```python
from build123d import *

# Parameters (mm, degrees)
SKETCH1_W                = 20
SKETCH1_H                = 10
BOSS_EXTRUDE1_DEPTH      = 3
SKETCH2_W                = 8
SKETCH2_H                = 9.5
BOSS_EXTRUDE2_DEPTH      = 6
BOSS_EXTRUDE3_DEPTH      = 6
BOSS_EXTRUDE3_DEPTH_BACK = 1.5
SKETCH3_R                = 6
CHAMFER1_SIZE            = 1
CHAMFER2_SIZE            = 1
CHAMFER3_SIZE            = 1
CHAMFER4_SIZE            = 2
CHAMFER5_SIZE            = 2
M2_CLEARANCE_HOLE1_D     = 2.4
SKETCH21_R               = 4.075
CUT_EXTRUDE10_DEPTH      = 6.5
SKETCH25_W               = 12
SKETCH25_H               = 4.5
BOSS_EXTRUDE6_DEPTH      = 3
M1_6_TAPPED_HOLE2_D      = 1.25
CUT_EXTRUDE15_START      = -3
SKETCH40_R               = 6
CUT_EXTRUDE15_DEPTH      = 3
BOSS_EXTRUDE8_START      = 1.7
SKETCH41_R               = 5
SKETCH41_R_2             = 4.075
BOSS_EXTRUDE8_DEPTH      = 1.7
CUT_EXTRUDE16_DEPTH      = 1


with BuildPart() as part:
    # Sketch1 → Boss-Extrude1 (new body)
    with BuildSketch(Plane.XY):
        Rectangle(SKETCH1_W, SKETCH1_H)
    extrude(amount=BOSS_EXTRUDE1_DEPTH)

    # Sketch2 → Boss-Extrude2 (add)
    with BuildSketch(Plane(origin=(0, 0, 0), x_dir=(-1, 0, 0), z_dir=(0, 0, -1))):
        with Locations((0, 4.75)):
            Rectangle(SKETCH2_W, SKETCH2_H)
    extrude(amount=BOSS_EXTRUDE2_DEPTH)

    # Sketch3 → Boss-Extrude3 (add, two sides: drawn at the far end of the back side and taken through both)
    with BuildSketch(Plane(origin=(0, 0, -6), x_dir=(-1, 0, 0), z_dir=(0, 0, -1)).offset(-BOSS_EXTRUDE3_DEPTH_BACK)):
        with Locations((0, 8.25)):
            Circle(SKETCH3_R)
    extrude(amount=BOSS_EXTRUDE3_DEPTH + BOSS_EXTRUDE3_DEPTH_BACK)

    # Chamfer1
    chamfer1_edges = [part.edges().sort_by_distance(p)[0] for p in [
        (-10, 5, 1.5),
        (10, 5, 1.5),
        (10, -5, 1.5),
        (-10, -5, 1.5),
    ]]
    chamfer(chamfer1_edges, length=CHAMFER1_SIZE)

    # Chamfer2
    chamfer2_edges = [part.edges().sort_by_distance(p)[0] for p in [
        (4, 2.5, 0),
        (-4, 2.5, 0),
        (0, 0, 0),
        (0, 0, -6),
    ]]
    chamfer(chamfer2_edges, length=CHAMFER2_SIZE)

    # Chamfer3
    # the kernel refuses this chamfer: 1 mm, written as the material it adds along each edge
    with BuildSketch(Plane(origin=(0, 8.25, -6), x_dir=(0.9161991076005935, -0.4007233400138756, 0), z_dir=(0.4007233400138756, 0.9161991076005935, 0))) as chamfer3_piece_1_section:
        Polygon((6 + CHAMFER3_SIZE, 0), (6, CHAMFER3_SIZE), (6, 0), align=None)
    chamfer3_piece_1 = revolve(axis=Axis((0, 8.25, -6), (0, 0, -1)), revolution_arc=132.753188511, mode=Mode.PRIVATE)
    chamfer3_piece_1 = split(chamfer3_piece_1, bisect_by=Plane(origin=(-4, 1.761901104, -6.488098896), z_dir=(1, 0, 0)), keep=Keep.TOP, mode=Mode.PRIVATE)
    chamfer3_piece_1 = split(chamfer3_piece_1, bisect_by=Plane(origin=(4, 1.761901104, -6.488098896), z_dir=(-1, 0, 0)), keep=Keep.TOP, mode=Mode.PRIVATE)
    add(chamfer3_piece_1)

    # Chamfer4
    chamfer4_edges = [part.edges().sort_by_distance(p)[0] for p in [
        (0, 5, 0),
    ]]
    chamfer(chamfer4_edges, length=CHAMFER4_SIZE)

    # Chamfer5
    # the kernel refuses this chamfer: 2 mm, written as the material it adds along each edge
    with BuildSketch(Plane(origin=(4, 5, -6.143365976), x_dir=(0.9996219169112968, -0.02749587661058651, 0), z_dir=(0, 0, 1))) as chamfer5_piece_1_section:
        Polygon((CHAMFER5_SIZE * 0.999621916911, CHAMFER5_SIZE * 0.0274958766106), (-CHAMFER5_SIZE * 0.0274958766106, CHAMFER5_SIZE * 0.999621916911), (0, 0), align=None)
    chamfer5_piece_1 = extrude(amount=13.286731952, mode=Mode.PRIVATE)
    chamfer5_piece_1 = split(chamfer5_piece_1, bisect_by=Plane(origin=(4.448565439, 5.872663391, -0.551434561), z_dir=(-0.7071067811865476, 0, 0.7071067811865476)), keep=Keep.TOP, mode=Mode.PRIVATE)
    chamfer5_piece_1 = split(chamfer5_piece_1, bisect_by=Plane(origin=(4.264786899, 6.620159706, 0.379840294), z_dir=(0, -0.7071067811865476, -0.7071067811865476)), keep=Keep.TOP, mode=Mode.PRIVATE)
    chamfer5_piece_1 = split(chamfer5_piece_1, bisect_by=Plane(origin=(4.264786899, 5.872663391, 0), z_dir=(0, 0, -1)), keep=Keep.TOP, mode=Mode.PRIVATE)
    add(chamfer5_piece_1)
    with BuildSketch(Plane(origin=(4, 5, -6.143365976), x_dir=(0.9996219169112968, -0.02749587661058651, 0), z_dir=(0, 0, 1))) as chamfer5_piece_2_section:
        Polygon((CHAMFER5_SIZE * 0.999621916911, CHAMFER5_SIZE * 0.0274958766106), (-CHAMFER5_SIZE * 0.0274958766106, CHAMFER5_SIZE * 0.999621916911), (0, 0), align=None)
    chamfer5_piece_2 = extrude(amount=13.286731952, mode=Mode.PRIVATE)
    chamfer5_piece_2 = split(chamfer5_piece_2, bisect_by=Plane(origin=(5.409489173, 5.195513982, 0.409489173), z_dir=(0.7071067811865476, 0, -0.7071067811865476)), keep=Keep.TOP, mode=Mode.PRIVATE)
    chamfer5_piece_2 = split(chamfer5_piece_2, bisect_by=Plane(origin=(5.545985564, 5.195513982, 0), z_dir=(0, 0, 1)), keep=Keep.TOP, mode=Mode.PRIVATE)
    add(chamfer5_piece_2)
    with BuildSketch(Plane(origin=(4, 5, -6.143365976), x_dir=(0.9996219169112968, -0.02749587661058651, 0), z_dir=(0, 0, 1))) as chamfer5_piece_3_section:
        Polygon((CHAMFER5_SIZE * 0.999621916911, CHAMFER5_SIZE * 0.0274958766106), (-CHAMFER5_SIZE * 0.0274958766106, CHAMFER5_SIZE * 0.999621916911), (0, 0), align=None)
    chamfer5_piece_3 = extrude(amount=13.286731952, mode=Mode.PRIVATE)
    chamfer5_piece_3 = split(chamfer5_piece_3, bisect_by=Plane(origin=(5.251928591, 5.490690976, 0.251928591), z_dir=(-0.7071067811865476, 0, 0.7071067811865476)), keep=Keep.TOP, mode=Mode.PRIVATE)
    chamfer5_piece_3 = split(chamfer5_piece_3, bisect_by=Plane(origin=(4.702100532, 5.844467162, 1.155532838), z_dir=(0, -0.7071067811865476, -0.7071067811865476)), keep=Keep.TOP, mode=Mode.PRIVATE)
    chamfer5_piece_3 = split(chamfer5_piece_3, bisect_by=Plane(origin=(4.702100532, 5.490690976, 0), z_dir=(0, 0, 1)), keep=Keep.TOP, mode=Mode.PRIVATE)
    add(chamfer5_piece_3)
    with BuildSketch(Plane(origin=(-4, 5, 7.143365976), x_dir=(-0.9996219169112968, -0.027495876610586487, 0), z_dir=(0, 0, -1))) as chamfer5_piece_4_section:
        Polygon((CHAMFER5_SIZE * 0.999621916911, CHAMFER5_SIZE * 0.0274958766106), (-CHAMFER5_SIZE * 0.0274958766106, CHAMFER5_SIZE * 0.999621916911), (0, 0), align=None)
    chamfer5_piece_4 = extrude(amount=13.286731952, mode=Mode.PRIVATE)
    chamfer5_piece_4 = split(chamfer5_piece_4, bisect_by=Plane(origin=(-5.251928591, 5.490690976, 0.251928591), z_dir=(0.7071067811865476, 0, 0.7071067811865476)), keep=Keep.TOP, mode=Mode.PRIVATE)
    chamfer5_piece_4 = split(chamfer5_piece_4, bisect_by=Plane(origin=(-4.702100532, 5.844467162, 1.155532838), z_dir=(0, -0.7071067811865476, -0.7071067811865476)), keep=Keep.TOP, mode=Mode.PRIVATE)
    chamfer5_piece_4 = split(chamfer5_piece_4, bisect_by=Plane(origin=(-4.702100532, 5.490690976, 0), z_dir=(0, 0, 1)), keep=Keep.TOP, mode=Mode.PRIVATE)
    add(chamfer5_piece_4)
    with BuildSketch(Plane(origin=(-4, 5, 7.143365976), x_dir=(-0.9996219169112968, -0.027495876610586487, 0), z_dir=(0, 0, -1))) as chamfer5_piece_5_section:
        Polygon((CHAMFER5_SIZE * 0.999621916911, CHAMFER5_SIZE * 0.0274958766106), (-CHAMFER5_SIZE * 0.0274958766106, CHAMFER5_SIZE * 0.999621916911), (0, 0), align=None)
    chamfer5_piece_5 = extrude(amount=13.286731952, mode=Mode.PRIVATE)
    chamfer5_piece_5 = split(chamfer5_piece_5, bisect_by=Plane(origin=(-4.448565439, 5.872663391, -0.551434561), z_dir=(0.7071067811865476, 0, 0.7071067811865476)), keep=Keep.TOP, mode=Mode.PRIVATE)
    chamfer5_piece_5 = split(chamfer5_piece_5, bisect_by=Plane(origin=(-4.264786899, 6.620159706, 0.379840294), z_dir=(0, -0.7071067811865476, -0.7071067811865476)), keep=Keep.TOP, mode=Mode.PRIVATE)
    chamfer5_piece_5 = split(chamfer5_piece_5, bisect_by=Plane(origin=(-4.264786899, 5.872663391, 0), z_dir=(0, 0, -1)), keep=Keep.TOP, mode=Mode.PRIVATE)
    add(chamfer5_piece_5)
    with BuildSketch(Plane(origin=(-4, 5, 7.143365976), x_dir=(-0.9996219169112968, -0.027495876610586487, 0), z_dir=(0, 0, -1))) as chamfer5_piece_6_section:
        Polygon((CHAMFER5_SIZE * 0.999621916911, CHAMFER5_SIZE * 0.0274958766106), (-CHAMFER5_SIZE * 0.0274958766106, CHAMFER5_SIZE * 0.999621916911), (0, 0), align=None)
    chamfer5_piece_6 = extrude(amount=13.286731952, mode=Mode.PRIVATE)
    chamfer5_piece_6 = split(chamfer5_piece_6, bisect_by=Plane(origin=(-5.409489173, 5.195513982, 0.409489173), z_dir=(-0.7071067811865476, 0, -0.7071067811865476)), keep=Keep.TOP, mode=Mode.PRIVATE)
    chamfer5_piece_6 = split(chamfer5_piece_6, bisect_by=Plane(origin=(-5.545985564, 5.195513982, 0), z_dir=(0, 0, 1)), keep=Keep.TOP, mode=Mode.PRIVATE)
    add(chamfer5_piece_6)

    # M2 Clearance Hole1 (through all)
    with Locations(Plane(origin=(0, 0, 0), x_dir=(-1, 0, 0), z_dir=(0, 0, -1))):
        with Locations((8, -3), (-8, -3)):
            Hole(M2_CLEARANCE_HOLE1_D / 2)

    # Sketch21 → Cut-Extrude10 (cut)
    with BuildSketch(Plane(origin=(0, 0, -12), x_dir=(-1, 0, 0), z_dir=(0, 0, -1))):
        with Locations((0, 8.25)):
            Circle(SKETCH21_R)
    extrude(amount=-CUT_EXTRUDE10_DEPTH, mode=Mode.SUBTRACT)

    # Sketch25 → Boss-Extrude6 (add)
    with BuildSketch(Plane.XY):
        with Locations((0, 7.25)):
            Rectangle(SKETCH25_W, SKETCH25_H)
    extrude(amount=BOSS_EXTRUDE6_DEPTH)

    # Sketch24 → CSK SLOT for M1.6 Countersunk Flat Head (revolve, cut)
    with BuildSketch(Plane(origin=(0, 8.25, 3), x_dir=(0, -1, 0), z_dir=(1, 0, 0))):
        Polygon((0, 0), (0, 40.540774557), (0.9, 40), (0.9, 9.9), (1.8, 9), (1.8, 0), align=None)
    revolve(axis=Axis((0, 8.25, 9.35), (0, 0, -1)), mode=Mode.SUBTRACT)

    # M1.6 Tapped Hole2 (through all)
    with Locations(Plane.ZY.offset(6)):
        with Locations((-7, 8.25)):
            Hole(M1_6_TAPPED_HOLE2_D / 2)

    # Sketch40 → Cut-Extrude15 (cut)
    with BuildSketch(Plane(origin=(0, 0, -12), x_dir=(-1, 0, 0), z_dir=(0, 0, -1)).offset(CUT_EXTRUDE15_START)):
        with Locations((0, 8.25)):
            Circle(SKETCH40_R)
    extrude(amount=CUT_EXTRUDE15_DEPTH, mode=Mode.SUBTRACT)

    # Sketch41 → Boss-Extrude8 (add)
    with BuildSketch(Plane(origin=(0, 0, -9), x_dir=(-1, 0, 0), z_dir=(0, 0, -1)).offset(BOSS_EXTRUDE8_START)):
        with Locations((0, 8.25)):
            Circle(SKETCH41_R)
        with Locations((0, 8.25)):
            Circle(SKETCH41_R_2, mode=Mode.SUBTRACT)
    extrude(amount=-BOSS_EXTRUDE8_DEPTH)

    # Sketch43 → Cut-Extrude16 (cut)
    with BuildSketch(Plane.XY.offset(-4.5)):
        with BuildLine():
            Line((-4, 9.5), (-1.295183385, 9.5))
            ThreePointArc((-1.295183385, 9.5), (0, 10.05), (1.295183385, 9.5))
            Line((1.295183385, 9.5), (4, 9.5))
            Line((4, 9.5), (5.868347297, 9.5))
            ThreePointArc((5.868347297, 9.5), (0, 14.25), (-5.868347297, 9.5))
            Line((-5.868347297, 9.5), (-4, 9.5))
        make_face()
    extrude(amount=-CUT_EXTRUDE16_DEPTH, mode=Mode.SUBTRACT)


solid = part.part
```
Geometry check sheet. Reference: the model listing, model coordinates, mm. A direction names the side the tool comes from. Coordinates: 2 decimals unless noted, no trailing zeros. Loops run counter-clockwise (first coordinate to the right, second up) from the corner with the lowest first, then second, coordinate; pieces in that order, holes last.
Item 1: Thickness scan on line 1 (Z direction, x = -5.1, y = 8.25) (3 decimals); line 2 (Y direction, x = -8, z = 2.3); line 3 (X direction, y = 8.25, z = -8.4) (3 decimals). Record the ranges inside material, lowest first.
Item 2: Sectioned sample at A-A, the plane y = -3. Record the boundary of the cut face in (x, z).
Item 3: Release check for a two-part mould opening along Y. For faces 5 (the face through (6.8, -2.95, 1.52)), 6 (the face through (-8, 5, 1)), 7 (the face through (0.1, 0.5, -5.5)), 8 (the face through (5.027, 8.672, -6.539)) record: released by +Y, released by -Y, zero draft, split by the parting line, or undercut.
Item 4: Go/stop test with flat-tipped pins: pin 1 Ø3.5 at (y, z) = (6, -5) entering from +X; pin 2 Ø1.5 at (y, z) = (7.5, -5.5) entering from -X; pin 3 Ø4 at (x, z) = (-1.5, -7.5) entering from +Y; pin 4 Ø1.7 at (x, y) = (1.5, 2) entering from -Z. Record where each tip stops, or that it passes through.
Item 5: Sectioned sample at C-C, the plane z = -0.25. Record the boundary of the cut face in (x, y), then the cut area to 3 significant figures.
Item 6: Sectioned sample at D-D, the plane y = 6.75. Record the boundary of the cut face in (x, z), then the cut area to 3 significant figures.
Item 7: Sectioned sample at B-B, the plane x = 8. Record the boundary of the cut face in (y, z).
Item 8: Access from +Z, -Z, +X, -X, +Y, -Y to the whole of each face (thin tool, end or side, straight path). Record for faces 1 (the face through (-3.764, 6.689, -8.136)), 2 (the face through (0, 13, -5.5)), 3 (the face through (0, 0, -3)), 4 (the face through (7, 5, 1)).
Check result:
1. line 1: z = -9 to -7.625, -6.375 to -4.5, 0 to 3
1. line 2: y = -5 to -4.2, -1.8 to 5
1. line 3: x = -6 to -4.075, 4.075 to 6
2. outline: (-10, 0) - (-9.2, 0) - (-9.2, 3) - (-10, 3) - close; (-6.8, 0) - (6.8, 0) - (6.8, 3) - (-6.8, 3) - close; (9.2, 0) - (10, 0) - (10, 3) - (9.2, 3) - close
3. face 5: undercut
3. face 6: released by +Y
3. face 7: released by -Y
3. face 8: undercut
4. pin 1: stops at x = 5.98
4. pin 2: stops at x = -6
4. pin 3: stops at y = 14.25
4. pin 4: stops at z = -9
5. outline: (-4.75, -0.75) - (4.75, -0.75) - (4.75, 6.25) - (4, 7) - (4, 9.5) - (1.3, 9.5) arc R1.8 cw (long way) to (-1.3, 9.5) - (-4, 9.5) - (-4, 7) - (-4.75, 6.25) - close
5. area: 83.9 mm2
6. outline: (-6, 0) - (-4.25, 0) - (-4.25, -0.75) - (-4, -1) - (-4, -4.5) - (-5.81, -4.5) - (-5.81, -9) - (-4.77, -9) - (-4.77, -10.7) - (-3.79, -10.7) - (-3.79, -5.5) - (-0.99, -5.5) - (-0.99, 3) - (-6, 3) - close; (0.99, -5.5) - (3.79, -5.5) - (3.79, -10.7) - (4.77, -10.7) - (4.77, -9) - (5.81, -9) - (5.81, -4.5) - (4, -4.5) - (4, -1) - (4.25, -0.75) - (4.25, 0) - (6, 0) - (6, 3) - (0.99, 3) - close
6. area: 84.6 mm2
7. outline: (-5, 0) - (-4.2, 0) - (-4.2, 3) - (-5, 3) - close; (-1.8, 0) - (5, 0) - (5, 3) - (-1.8, 3) - close
8. face 1: -Z
8. face 2: +Z, +X, -X, +Y
8. face 3: -Z, +X, -X, -Y
8. face 4: +Z, -Z, +X, +Y
